Autodesk Inventor part; units mm, degrees
ref_plane "YZ Plane" through (0, 0, 0) normal (1, 0, 0) x (0, 1, 0)
ref_plane "XZ Plane" through (0, 0, 0) normal (0, 1, 0) x (-1, 0, 0)
ref_plane "XY Plane" through (0, 0, 0) normal (0, 0, 1) x (1, 0, 0)
sketch "Sketch1" plane through (0, 0, 0) normal (0, 0, 1) x (1, 0, 0)
  line L0 (-62.4, 25.45) -> (62.4, 25.45)
  line L1 (62.4, 25.45) -> (62.4, -25.45)
  line L2 (62.4, -25.45) -> (-62.4, -25.45)
  line L3 (-62.4, -25.45) -> (-62.4, 25.45)
  point P0 (0, 0)
  dimension "d0" = 124.8
  dimension "d1" = 50.9
  dimension "d2" = 62.4
  dimension "d3" = 25.45
extrude "Extrusion1" add sketch "Sketch1" along normal blind 10.0076
fillet "Fillet1" radius 3.175 1 edges at (-62.4, 25.45, 5.0038)
fillet "Fillet2" radius 3.175 3 edges at (62.4, 25.45, 5.0038) (62.4, -25.45, 5.0038) (-62.4, -25.45, 5.0038)
sketch "Sketch6" plane through (0, 0, 10.0076) normal (0, 0, 1) x (1, 0, 0)
  arc A0 (10.55, -12.337) -> (15.55, -7.337) centre (10.55, -7.337) ccw
  line L0 (15.55, -7.337) -> (15.55, 5.963)
  arc A1 (15.55, 5.963) -> (10.55, 10.963) centre (10.55, 5.963) ccw
  line L1 (10.55, 10.963) -> (-10.55, 10.963)
  arc A2 (-10.55, 10.963) -> (-15.55, 5.963) centre (-10.55, 5.963) ccw
  line L2 (-15.55, 5.963) -> (-15.55, -7.337)
  arc A3 (-15.55, -7.337) -> (-10.55, -12.337) centre (-10.55, -7.337) ccw
  line L3 (-10.55, -12.337) -> (10.55, -12.337)
  circle A4 centre (-20, -0.687) radius 1.8
  circle A5 centre (20, -0.687) radius 1.8
  point P0 (0, 0)
extrude "Extrusion7" cut sketch "Sketch6" against normal up to surface (10.0076 mm away)
properties part number "front cover"
Can you work these out from the model? Positions are in its coordinate system, mm. A direction names the side the tool comes from. Coordinates: 2 decimals unless noted, no trailing zeros. Write each loop counter-clockwise with the first axis right and the second up, starting at its lowest first coordinate (ties: lowest second). Pieces come first, ordered by that corner, then holes.
Q1. Please list where these lines run through material, in increasing order: L1, parallel to Y at x = -20, z = 6.75; L2, parallel to X at y = 5, z = 9.5; L3, parallel to Y at x = 4, z = 4.
Results found:
L1: y = -25.45 to -2.49, 1.11 to 25.45
L2: x = -62.4 to -15.55, 15.55 to 62.4
L3: y = -25.45 to -12.34, 10.96 to 25.45
Q2. Imagine slicing it at A-A, the plane x = 20. List the corners of the cut face in (y, z) for me, plus the area to 3 significant figures.
Results found:
outline: (-25.45, 0) - (-2.49, 0) - (-2.49, 10.01) - (-25.45, 10.01) - close; (1.11, 0) - (25.45, 0) - (25.45, 10.01) - (1.11, 10.01) - close
area: 473 mm2
Q3. Imagine slicing it at B-B, the plane z = 1.75. List the corners of the cut face in (x, y) for me (3 decimals), plus the area to 3 significant figures.
Results found:
outline: (-62.4, -22.275) arc R3.175 ccw to (-59.225, -25.45) - (59.225, -25.45) arc R3.175 ccw to (62.4, -22.275) - (62.4, 22.275) arc R3.175 ccw to (59.225, 25.45) - (-59.225, 25.45) arc R3.175 ccw to (-62.4, 22.275) - close; hole circle Ø3.6 at (-20, -0.687); hole (-15.55, -7.337) arc R5 ccw to (-10.55, -12.337) - (10.55, -12.337) arc R5 ccw to (15.55, -7.337) - (15.55, 5.963) arc R5 ccw to (10.55, 10.963) - (-10.55, 10.963) arc R5 ccw to (-15.55, 5.963) - close; hole circle Ø3.6 at (20, -0.687)
area: 5,620 mm2
Q4. If we mould it in two halves opening along X, with no side actions, what happens to faces 3 (the face through (14.124, 9.459, 5.074)), 4 (the face through (-61.45, 24.54, 5.07)), 5 (the face through (14.05, -10.91, 5.07)), 6 (the face through (-1, 25.45, 5))? For each: +X half, -X half, draft (parallel to the pull), parting line (faces both ways), or undercut.
Results found:
face 3: undercut
face 4: -X half
face 5: undercut
face 6: draft
Q5. Which directions (+Z, -Z, +X, -X, +Y, -Y) give clear straight access to the entire face, cutting with the end or side of a thin tool? Please do faces 1 (the face through (-14.124, -10.833, 5.074)), 2 (the face through (61.49, 24.5, 5.07)).
Results found:
face 1: +Z, -Z
face 2: +Z, -Z, +X, +Y
Q6. For P1, Ø2, axis at x = -20, y = -0.687, coming from the +Z side, with a flat end and sliding along its axis, tell me the tip position at first contact or that it passes through.
Results found:
P1: passes through
